Could you check a few things on this model? Use its own coordinates, in mm. A direction names the side the tool comes from. Give positions to 0.01 mm unless a question says otherwise; leave off trailing zeros. Loops run counter-clockwise (first coordinate to the right, second up) from the corner with the lowest first, then second, coordinate; pieces in that order, holes last. Notation, with made-up numbers: (-20, 16.5) - (27, 16.5) arc R26 cw to (27, 50.5) - close; hole circle Ø4 at (30, -25.5). An arc over 180 degrees is marked (long way). One line per item, written item: value. Start each with the question number.
Q1. I want a section at B-B (z = -53). Please give me the cut outline in (x, y).
Q2. I'm going to push flat-ended pins straight in: P1, Ø4, axis at x = -23, y = 1, coming from the +Z side; P2, Ø6, axis at y = -23, z = -53, coming from the -X side; P3, Ø1, axis at x = 25.5, y = 23, coming from the -Z side. Where does each tip first touch, or does it pass through?
Q3. I want a section at D-D (y = 1). Please give me the cut outline in (x, z).
Q4. I want a section at C-C (x = 0). Please give me the cut outline in (y, z), then the cut area to 3 significant figures.
Q5. If we mould it in two halves opening along Z, with no side actions, what happens to faces 1 (the face through (0, 16, 5)), 2 (the face through (32.53, 25.11, -54.34)), 3 (the face through (-0.33, -27.48, 2.46))? For each: released by +Z, released by -Z, zero draft, split by the parting line, or undercut.
Q6. If I drill on line 1 (Z direction, x = 31.6, y = -23); line 2 (Y direction, x = 0, z = 4); line 3 (Y direction, x = 32.6, z = -53), over which ranges is the centre line in solid material (lowest first)? Write a range as from..to.
Q7. For faces 4 (the face through (15, 35, 1)), 5 (the face through (-17, 0, 0)), which set-ups out of +Z, -Z, +X, -X, +Y, -Y let a thin tool reach every point of the face, with its end or its side?
Q8. I want a section at A-A (y = -12). Please give me the cut outline in (x, z), then the cut area to 3 significant figures.
Autodesk Inventor part; units mm, degrees
ref_plane "YZ Plane" through (0, 0, 0) normal (1, 0, 0) x (0, 1, 0)
ref_plane "XZ Plane" through (0, 0, 0) normal (0, 1, 0) x (-1, 0, 0)
ref_plane "XY Plane" through (0, 0, 0) normal (0, 0, 1) x (1, 0, 0)
sketch "Sketch1" plane through (0, 0, 0) normal (0, 0, 1) x (1, 0, 0)
  line L0 (-35, 35) -> (35, 35)
  line L1 (35, 35) -> (35, -35)
  line L2 (35, -35) -> (-35, -35)
  line L3 (-35, -35) -> (-35, 35)
  line L4 (-35, 35) -> (35, -35) construction
  line L5 (35, 35) -> (-35, -35) construction
  circle A0 centre (0, 0) radius 15
  circle A1 centre (0, 0) radius 25
  circle A2 centre (-25, 0) radius 2.5
  circle A3 centre (0, -25) radius 2.5
  circle A4 centre (25, 0) radius 2.5
  circle A5 centre (0, 25) radius 2.5
  dimension "d3" = 50
  dimension "d0" = 70
  dimension "d1" = 70
  dimension "d2" = 30
  dimension "d4" = 5
  dimension "d7" = 360
extrude "Extrusion1" add sketch "Sketch1" along normal blind 5 contours L0 L1 L2 L3 | A4 A1 A3 A2 A5
sketch "Sketch2" plane through (35, -35, 0) normal (1, 0, 0) x (0, 0, -1)
  line L0 (-5, 0) -> (-5, 70)
  line L1 (-5, 70) -> (65, 70)
  line L2 (65, 70) -> (65, 0)
  line L3 (65, 0) -> (-5, 0)
  line L4 (-5, 0) -> (-5, 70)
  point P0 (0, 35)
  dimension "d11" = 70
  dimension "d12" = 70
extrude "Extrusion2" add sketch "Sketch2" against normal blind 5
sketch "Sketch3" plane through (35, -35, 5) normal (1, 0, 0) x (0, 0, -1)
  line L0 (70, 70) -> (0, 70)
  line L1 (0, 0) -> (0, 70)
  line L2 (70, 0) -> (0, 0)
  line L3 (70, 0) -> (70, 70)
  line L4 (12, 58) -> (58, 58)
  line L5 (58, 58) -> (58, 12)
  line L6 (58, 12) -> (12, 12)
  line L7 (12, 12) -> (12, 58)
  circle A0 centre (12, 58) radius 2.5
  circle A1 centre (58, 58) radius 2.5
  circle A2 centre (12, 12) radius 2.5
  circle A3 centre (58, 12) radius 2.5
  point P0 (5, 35)
  dimension "d15" = 12
  dimension "d16" = 5
  dimension "d19" = 46
  dimension "d22" = 46
extrude "Extrusion3" cut sketch "Sketch3" against normal blind 5 contours L7 A0 L4 | L4 A0 L7 | A1 L5 L4 | L4 L5 A1 | A2 L6 L7 | L7 L6 A2 | A3 L6 L5 | L5 L6 A3
properties part number "SOPORTE DE MOTOR"
Worked answers:
1. outline: (30, -35) - (35, -35) - (35, -25.5) - (30, -25.5) - close; (30, -20.5) - (35, -20.5) - (35, 20.5) - (30, 20.5) - close; (30, 25.5) - (35, 25.5) - (35, 35) - (30, 35) - close
2. P1: stops at z = 5
2. P2: stops at x = 30
2. P3: stops at z = 0
3. outline: (-35, 0) - (-27.29, 0) - (-27.29, 5) - (-35, 5) - close; (-22.71, 0) - (-14.97, 0) - (-14.97, 5) - (-22.71, 5) - close; (14.97, 0) - (22.71, 0) - (22.71, 5) - (14.97, 5) - close; (27.29, 0) - (30, 0) - (30, -65) - (35, -65) - (35, 5) - (27.29, 5) - close
4. outline: (-35, 0) - (-27.5, 0) - (-27.5, 5) - (-35, 5) - close; (-22.5, 0) - (-15, 0) - (-15, 5) - (-22.5, 5) - close; (15, 0) - (22.5, 0) - (22.5, 5) - (15, 5) - close; (27.5, 0) - (35, 0) - (35, 5) - (27.5, 5) - close
4. area: 150 mm²
5. face 1: released by +Z
5. face 2: undercut
5. face 3: zero draft
6. line 1: z = -65..-55.5, -50.5..-9.5, -4.5..5
6. line 2: y = -35..-27.5, -22.5..-15, 15..22.5, 27.5..35
6. line 3: y = -35..-25.5, -20.5..20.5, 25.5..35
7. face 4: +Z, -Z, +X, -X, +Y
7. face 5: -Z, -X, +Y, -Y
8. outline: (-35, 0) - (-9, 0) - (-9, 5) - (-35, 5) - close; (9, 0) - (30, 0) - (30, -65) - (35, -65) - (35, 5) - (9, 5) - close
8. area: 585 mm²
